from build123d import *

# Parameters (mm, degrees)
SKETCH2_W          = 50
SKETCH2_H          = 5
FILLET2_R          = 2.5
SKETCH3_R          = 5
CUT_EXTRUDE1_DEPTH = 50
FILLET3_R          = 7.5


with BuildPart() as part:
    # Sweep1: sweep along a path in Sketch1
    with BuildLine(Plane(origin=(0, 0, 0), x_dir=(0, 0, -1), z_dir=(1, 0, 0))) as sweep1_path:
        Line((0, 0), (22.5, 0))
        Line((22.5, 0), (22.5, -67.5))
        ThreePointArc((22.5, -67.5), (40, -85), (57.5, -67.5))
        Line((57.5, -67.5), (57.5, -30))
        Line((57.5, -30), (80, -30))
    # Sketch2 → Sweep1 (sweep)
    with BuildSketch(Plane.XY):
        Rectangle(SKETCH2_W, SKETCH2_H)
    sweep(path=sweep1_path.line, transition=Transition.RIGHT)

    # Fillet2
    fillet2_edges = [part.edges().sort_by_distance(p)[0] for p in [
        (0, 2.5, -25),
        (0, -2.5, -20),
        (0, -27.5, -55),
        (0, -32.5, -60),
    ]]
    fillet(fillet2_edges, radius=FILLET2_R)

    # Sketch3 → Cut-Extrude1 (cut)
    with BuildSketch(Plane(origin=(0, 2.5, 0), x_dir=(1, 0, 0), z_dir=(0, 1, 0))):
        with Locations((-15, 70)):
            Circle(SKETCH3_R)
        with Locations((15, 70)):
            Circle(SKETCH3_R)
        with Locations((15, 10)):
            Circle(SKETCH3_R)
        with Locations((-15, 10)):
            Circle(SKETCH3_R)
    extrude(amount=-CUT_EXTRUDE1_DEPTH, mode=Mode.SUBTRACT)

    # Fillet3
    fillet3_edges = [part.edges().sort_by_distance(p)[0] for p in [
        (25, 0, 0),
        (-25, -30, -80),
        (25, -30, -80),
        (-25, 0, 0),
    ]]
    fillet(fillet3_edges, radius=FILLET3_R)


solid = part.part
Verification items for the finished model (mm, model axes). A direction names the side the tool comes from. Coordinates: 2 decimals unless noted, no trailing zeros. Order: outer loops, then holes, each group sorted by start corner. A loop starts at its lowest first (then second) coordinate and runs counter-clockwise, first axis right, second up. Notation, with made-up numbers: (40, 56.25) -> (62, 56.25) arc R27 ccw to (62, 84.25) -> close; hole circle Ø4 at (-33, 3.5). An arc over 180 degrees is marked (long way). Put each result on its own line as item: value. Start each with the question number.
1. Cross-section at C-C, the plane z = -10. Record the boundary of the cut face in (x, y).
2. Go/stop test with flat-tipped pins: pin 1 Ø18 at (x, z) = (11.5, -71) entering from +Y; pin 2 Ø9 at (x, z) = (9.5, -5.5) entering from -Y; pin 3 Ø15 at (x, y) = (-3, -46) entering from -Z; pin 4 Ø8 at (y, z) = (-26.5, -54) entering from -X. Record where each tip stops, or that it passes through.
3. Material ranges on L1, parallel to X at y = 0, z = -10; L2, parallel to Z at x = 4, y = -47; L3, parallel to Z at x = -15, y = -28.5, recorded low to high. Write a range as [from, to].
4. Access from +Z, -Z, +X, -X, +Y, -Y to the whole of each face (thin tool, end or side, straight path). Record for faces 1 (the flat face through (0, -34, -25)), 2 (the flat face through (0, -2.5, -9)), 3 (the flat face through (0, 2.5, -11)).
5. Cross-section at B-B, the plane x = 15. Record the boundary of the cut face in (y, z), then the cut area to 3 significant figures.
6. Mould release check, pull along Z, two halves, no side actions. Record for faces 4 (the flat face through (0, -32.5, -71)), 5 (the flat face through (0, -48, -55)), 6 (the cylindrical face through (0, 2, -24)): released by +Z, released by -Z, zero draft, split by the parting line, or undercut.
7. Cross-section at A-A, the plane y = -41. Record the boundary of the cut face in (x, z).
8. Cross-section at D-D, the plane y = -77. Record the boundary of the cut face in (x, z), then the cut area to 3 significant figures.
Computed:
1. outline: (-25, -2.5) -> (-20, -2.5) -> (-20, 2.5) -> (-25, 2.5) -> close; (-10, -2.5) -> (10, -2.5) -> (10, 2.5) -> (-10, 2.5) -> close; (20, -2.5) -> (25, -2.5) -> (25, 2.5) -> (20, 2.5) -> close
2. pin 1: y = -27.5
2. pin 2: y = -2.5
2. pin 3: z = -60
2. pin 4: x = -25
3. L1: [-25, -20], [-10, 10], [20, 25]
3. L2: [-60, -55], [-25, -20]
3. L3: [-80, -75], [-65, -55.5], [-25, -20]
4. face 1: +X, -X, +Y
4. face 2: +Z, +X, -X, -Y
4. face 3: +Z, -Z, +X, -X, +Y
5. outline: (-67.5, -60) -> (-35, -60) arc R2.5 cw to (-32.5, -62.5) -> (-32.5, -65) -> (-27.5, -65) -> (-27.5, -57.5) arc R2.5 ccw to (-30, -55) -> (-67.5, -55) arc R15 cw to (-67.5, -25) -> (0, -25) arc R2.5 ccw to (2.5, -22.5) -> (2.5, -15) -> (-2.5, -15) -> (-2.5, -17.5) arc R2.5 cw to (-5, -20) -> (-67.5, -20) arc R20 ccw to start; (-32.5, -80) -> (-27.5, -80) -> (-27.5, -75) -> (-32.5, -75) -> close; (-2.5, -5) -> (2.5, -5) -> (2.5, 0) -> (-2.5, 0) -> close
5. area: 925 mm2
6. face 4: zero draft
6. face 5: undercut
6. face 6: released by -Z
7. outline: (-25, -60) -> (25, -60) -> (25, -55) -> (-25, -55) -> close; (-25, -25) -> (25, -25) -> (25, -20) -> (-25, -20) -> close
8. outline: (-25, -57.6) -> (25, -57.6) -> (25, -51.61) -> (-25, -51.61) -> close; (-25, -28.39) -> (25, -28.39) -> (25, -22.4) -> (-25, -22.4) -> close
8. area: 599 mm2
